Design review of the part built by this model. Coordinates are the model's own, in mm. Give positions to 0.01 mm unless a question says otherwise; leave off trailing zeros. Order: outer loops, then holes, each group sorted by start corner. A loop starts at its lowest first (then second) coordinate and runs counter-clockwise, first axis right, second up.
```python
from build123d import *

# Parameters (mm, degrees)
F1_DEPTH = 2706
F2_R     = 2
F3_R     = 1


with BuildPart() as f1:
    # F0 (on Top) → F1 (new body)
    with BuildSketch(Plane.XY):
        Polygon((20, 10), (-20, 10), (-20, -5), (-17, -5), (-17, 7), (-2, 7), (-2, -9.5), (-8.5, -9.5), (-8.5, -12.5), (0, -12.5), (8.5, -12.5), (8.5, -9.5), (2, -9.5), (2, 7), (17, 7), (17, -5), (20, -5), align=None)
    extrude(amount=F1_DEPTH)

    # F2
    f2_edges = [f1.edges().sort_by_distance(p)[0] for p in [
        (-20, 10, 1353),
        (20, 10, 1353),
    ]]
    fillet(f2_edges, radius=F2_R)

    # F3
    f3_edges = [f1.edges().sort_by_distance(p)[0] for p in [
        (-17, -5, 1353),
        (-20, -5, 1353),
        (-17, 7, 1353),
        (2, 7, 1353),
        (17, -5, 1353),
        (20, -5, 1353),
        (8.5, -9.5, 1353),
        (8.5, -12.5, 1353),
        (-8.5, -12.5, 1353),
        (-8.5, -9.5, 1353),
        (-2, -9.5, 1353),
        (-2, 7, 1353),
        (17, 7, 1353),
        (2, -9.5, 1353),
    ]]
    fillet(f3_edges, radius=F3_R)


solid = f1.part
```
1. For line 1 along X through (y, z) = (5.25, 1744); line 2 along Y through (x, z) = (-5.5, 1372); line 3 along Y through (x, z) = (18.5, 1558.5), list the stretches that pass through material, from the lowest coordinate up.
Recorded:
line 1: x = -20 to -17, -2 to 2, 17 to 20
line 2: y = -12.5 to -9.5, 7 to 10
line 3: y = -5 to 9.94
2. For pin 1 (0.8 mm diameter, centred on y = -11, z = 1180, fed in from -X); pin 2 (1.1 mm diameter, centred on x = 18.5, z = 848.5, fed in from -Y); pin 3 (8 mm diameter, centred on x = 13.5, z = 677.5, fed in from -Y), all flat-tipped, find the tip position at first contact; note any pin that passes through.
Recorded:
pin 1: stops at x = -8.5
pin 2: stops at y = -5
pin 3: stops at y = -4.87
3. Take a section at A-A (y = 2.5). State the section outline as (x, z) points, then the cut area to 3 significant figures.
Recorded:
outline: (-20, 0) - (-17, 0) - (-17, 2706) - (-20, 2706) - close; (-2, 0) - (2, 0) - (2, 2706) - (-2, 2706) - close; (17, 0) - (20, 0) - (20, 2706) - (17, 2706) - close
area: 27,100 mm2
